from build123d import *

# Parameters (mm, degrees)
SKETCH1_W               = 671.5125
SKETCH1_H               = 299.466
BOSS_EXTRUDE1_DEPTH     = 9.525
BOSS_EXTRUDE2_DEPTH     = 19.05
FILLET1_R               = 25.4
SKETCH3_R               = 17.5
SKETCH3_R_2             = 14.2875
CUT_EXTRUDE1_DEPTH      = 1
CUT_EXTRUDE1_DEPTH_BACK = 20.05
CUT_EXTRUDE2_DEPTH      = 7.9375
CUT_EXTRUDE3_DEPTH      = 409.263892457
CUT_EXTRUDE3_DEPTH_BACK = 409.263892457
CUT_EXTRUDE5_START      = -19.05
SKETCH3_3_R             = 3.96875
CUT_EXTRUDE5_DEPTH      = 11.1125
SKETCH8_R               = 5.953125
CUT_EXTRUDE6_DEPTH      = 1.016


with BuildPart() as part:
    # Sketch1 → Boss-Extrude1 (new body, symmetric)
    with BuildSketch(Plane(origin=(0, 0, 0), x_dir=(1, 0, 0), z_dir=(0, 1, 0))):
        Rectangle(SKETCH1_W, SKETCH1_H)
    extrude(amount=BOSS_EXTRUDE1_DEPTH, both=True)

    # Sketch2 → Boss-Extrude2 (add)
    with BuildSketch(Plane(origin=(0, 9.525, 0), x_dir=(1, 0, 0), z_dir=(0, 1, 0))):
        Polygon((335.75625, -149.733), (374.643853371, -149.733), (412.08325, 116.6621492), (335.75625, 116.6621492), align=None)
        Polygon((-335.75625, 116.6621492), (-335.75625, -149.733), (-374.643853371, -149.733), (-412.08325, 116.6621492), align=None)
    extrude(amount=-BOSS_EXTRUDE2_DEPTH)

    # Fillet1
    fillet1_edges = [part.edges().sort_by_distance(p)[0] for p in [
        (374.643853371, 0, 149.733),
        (412.08325, 0, -116.6621492),
        (-412.08325, 0, -116.6621492),
        (-374.643853371, 0, 149.733),
    ]]
    fillet(fillet1_edges, radius=FILLET1_R)

    # Sketch3 → Cut-Extrude1 (cut, two sides)
    with BuildSketch(Plane(origin=(0, 9.525, 0), x_dir=(1, 0, 0), z_dir=(0, 1, 0))) as cut_extrude1_sk:
        with Locations((-275.836957508, -19.05)):
            Circle(SKETCH3_R)
        with Locations((-180.836957508, 7.95)):
            Circle(SKETCH3_R_2)
        with Locations((-145.836957508, 16.95)):
            Circle(SKETCH3_R_2)
        with Locations((-145.836957508, -19.05)):
            Circle(SKETCH3_R_2)
        with Locations((-180.836957508, -28.05)):
            Circle(SKETCH3_R_2)
        with Locations((-212.086957508, -10.05)):
            Circle(SKETCH3_R_2)
        with Locations((-212.086957508, -46.05)):
            Circle(SKETCH3_R_2)
        with Locations((-212.086957508, 82.55)):
            Circle(SKETCH3_R_2)
        with Locations((-164.36967051, 82.55)):
            Circle(SKETCH3_R_2)
        with Locations((130.563042492, -19.05)):
            Circle(SKETCH3_R)
        with Locations((225.563042492, 7.95)):
            Circle(SKETCH3_R_2)
        with Locations((260.563042492, 16.95)):
            Circle(SKETCH3_R_2)
        with Locations((260.563042492, -19.05)):
            Circle(SKETCH3_R_2)
        with Locations((225.563042492, -28.05)):
            Circle(SKETCH3_R_2)
        with Locations((194.313042492, -10.05)):
            Circle(SKETCH3_R_2)
        with Locations((194.313042492, -46.05)):
            Circle(SKETCH3_R_2)
        with Locations((194.313042492, 82.55)):
            Circle(SKETCH3_R_2)
        with Locations((242.03032949, 82.55)):
            Circle(SKETCH3_R_2)
        with Locations((-44.45, 57.15)):
            Circle(SKETCH3_R_2)
        with Locations((0, 57.15)):
            Circle(SKETCH3_R_2)
        with Locations((44.45, 57.15)):
            Circle(SKETCH3_R_2)
    extrude(amount=CUT_EXTRUDE1_DEPTH, mode=Mode.SUBTRACT)
    extrude(cut_extrude1_sk.sketch, amount=-CUT_EXTRUDE1_DEPTH_BACK, mode=Mode.SUBTRACT)

    # Sketch4 → Cut-Extrude2 (cut)
    with BuildSketch(Plane.XZ.offset(9.525)):
        with BuildLine():
            Line((-355.727, -48.520132908), (-355.727, 91.179867092))
            ThreePointArc((-355.727, 91.179867092), (-346.075, 100.831867092), (-336.423, 91.179867092))
            Line((-336.423, 91.179867092), (-336.423, -48.520132908))
            ThreePointArc((-336.423, -48.520132908), (-346.075, -58.172132908), (-355.727, -48.520132908))
        make_face()
        with BuildLine():
            Line((355.727, -48.520132908), (355.727, 91.179867092))
            ThreePointArc((355.727, 91.179867092), (346.075, 100.831867092), (336.423, 91.179867092))
            Line((336.423, 91.179867092), (336.423, -48.520132908))
            ThreePointArc((336.423, -48.520132908), (346.075, -58.172132908), (355.727, -48.520132908))
        make_face()
    extrude(amount=-CUT_EXTRUDE2_DEPTH, mode=Mode.SUBTRACT)

    # Sketch5 → Cut-Extrude3 (cut, two sides)
    with BuildSketch(Plane(origin=(0, 0, 0), x_dir=(0, 0, -1), z_dir=(1, 0, 0))) as cut_extrude3_sk:
        Polygon((132.550024206, 9.525), (131.232981568, 6.35), (124.767204191, 9.032111651), (126.084246829, 12.207111651), align=None)
    extrude(amount=CUT_EXTRUDE3_DEPTH, mode=Mode.SUBTRACT)
    extrude(cut_extrude3_sk.sketch, amount=-CUT_EXTRUDE3_DEPTH_BACK, mode=Mode.SUBTRACT)

    # Sketch3<3> → Cut-Extrude5 (cut)
    with BuildSketch(Plane(origin=(0, 9.525, 0), x_dir=(1, 0, 0), z_dir=(0, 1, 0)).offset(CUT_EXTRUDE5_START)):
        with Locations((-308.636957508, 18.9)):
            Circle(SKETCH3_3_R)
        with Locations((-243.036957508, 18.9)):
            Circle(SKETCH3_3_R)
        with Locations((-308.636957508, -57)):
            Circle(SKETCH3_3_R)
        with Locations((-243.036957508, -57)):
            Circle(SKETCH3_3_R)
        with Locations((97.763042492, 18.9)):
            Circle(SKETCH3_3_R)
        with Locations((163.363042492, 18.9)):
            Circle(SKETCH3_3_R)
        with Locations((97.763042492, -57)):
            Circle(SKETCH3_3_R)
        with Locations((163.363042492, -57)):
            Circle(SKETCH3_3_R)
    extrude(amount=CUT_EXTRUDE5_DEPTH, mode=Mode.SUBTRACT)

    # Sketch8 → Cut-Extrude6 (cut)
    with BuildSketch(Plane.XZ.offset(9.525)):
        with Locations((163.363042492, -18.9)):
            Circle(SKETCH8_R)
        with Locations((163.363042492, 57)):
            Circle(SKETCH8_R)
        with Locations((97.763042492, 57)):
            Circle(SKETCH8_R)
        with Locations((97.763042492, -18.9)):
            Circle(SKETCH8_R)
        with Locations((-243.036957508, -18.9)):
            Circle(SKETCH8_R)
        with Locations((-243.036957508, 57)):
            Circle(SKETCH8_R)
        with Locations((-308.636957508, 57)):
            Circle(SKETCH8_R)
        with Locations((-308.636957508, -18.9)):
            Circle(SKETCH8_R)
    extrude(amount=-CUT_EXTRUDE6_DEPTH, mode=Mode.SUBTRACT)


solid = part.part
Design review of the part built by this model. Coordinates are the model's own, in mm. A direction names the side the tool comes from. Round coordinates to 2 decimals unless told otherwise and drop trailing zeros. One line per question, with ' | ' between items.
(1) Insertion check: P1, Ø6.5, axis at y = -4, z = 44.5, coming from the +X side; P2, Ø5.5, axis at y = -1, z = -135, coming from the +X side; P3, Ø3.5, axis at x = 95, z = 55, coming from the -Y side. Each pin has a flat end and moves straight along its axis. Give the tip position at first contact, or say it passes through.
Result sheet:
P1: x = 389.89 | P2: x = 335.76 | P3: y = -8.51
(2) Machinability: for faces 1 (the cylindrical face through (230.69, 0.13, -73.86)), 2 (the flat face through (335.756, 0, -133)), 3 (the flat face through (-335.756, 0, -133)), which of the approach directions +Z, -Z, +X, -X, +Y, -Y give a long, thin tool a straight path to every point of the face, cutting with its end or side? Answer none if there is none.
Result sheet:
face 1: +Y, -Y | face 2: -Z, +X, +Y, -Y | face 3: -Z, -X, +Y, -Y
(3) Wall thickness on line 1 (Z direction, x = 260, y = -7); line 2 (Z direction, x = 198, y = -2.5); line 3 (X direction, y = 7.5, z = -95.5): over which ranges is each line inside the solid? List them lowest first. Write a range as [from, to].
Result sheet:
line 1: [-149.73, -31.23], [-2.67, 4.77], [33.33, 149.73] | line 2: [-149.73, -96.35], [-68.75, -3.75], [23.85, 32.25], [59.85, 149.73] | line 3: [-407.91, -218.12], [-206.05, -170.41], [-158.33, 188.28], [200.35, 235.99], [248.07, 407.91]
(4) Draft analysis for pull direction X (two halves, no side actions). For faces 4 (the flat face through (-346, -1.588, 22)), 5 (the flat face through (392.655, 0.133, 21.58)), 6 (the flat face through (-392.655, 0.133, 21.58)), state which applies: released by +X, released by -X, zero draft, split by the parting line, or undercut.
Result sheet:
face 4: undercut | face 5: released by +X | face 6: released by -X
